from build123d import *

# Parameters (mm, degrees)
SKETCH_1_R          = 13.5
EXTRUDE_1_DEPTH     = 10
SKETCH_2_W          = 12
SKETCH_2_H          = 60
EXTRUDE_2_DEPTH     = 10
SKETCH_3_R          = 10.25
CUT_EXTRUDE_1_DEPTH = 10


with BuildPart() as part:
    # 草图1 → 凸台-拉伸1 (new body)
    with BuildSketch(Plane(origin=(0, 0, 0), x_dir=(1, 0, 0), z_dir=(0, 1, 0))):
        with Locations(Location((0, 0, 0), (0, 0, 270))):
            Circle(SKETCH_1_R)
    extrude(amount=EXTRUDE_1_DEPTH)

    # 草图2 → 凸台-拉伸2 (add)
    with BuildSketch(Plane(origin=(0, 10, 0), x_dir=(1, 0, 0), z_dir=(0, 1, 0))):
        Rectangle(SKETCH_2_W, SKETCH_2_H)
    extrude(amount=-EXTRUDE_2_DEPTH)

    # 草图3 → 切除-拉伸1 (cut)
    with BuildSketch(Plane(origin=(0, 10, 0), x_dir=(1, 0, 0), z_dir=(0, 1, 0))):
        with Locations(Location((0, 0, 0), (0, 0, 270))):
            Circle(SKETCH_3_R)
    extrude(amount=-CUT_EXTRUDE_1_DEPTH, mode=Mode.SUBTRACT)


solid = part.part
The listing builds one solid part. Answer for the finished solid, in the listing's coordinates (mm). A direction names the side the tool comes from. Coordinates: 2 decimals unless noted, no trailing zeros. Order: outer loops, then holes, each group sorted by start corner. A loop starts at its lowest first (then second) coordinate and runs counter-clockwise, first axis right, second up. Notation, with made-up numbers: M 88,67.5 L 115,67.5 A28 cw 115,91.5 Z; hole C -21,-3.75 d4. An arc over 180 degrees is marked long. Use CSV: the item, a comma, the result in double quotes.
Q1. Section A-A (y = 8) is taken. Determine the outline of the cut face in (x, z), then the cut area to 4 significant figures.
Here are the results:
outline,"M -6,-30 L 6,-30 L 6,-12.09 A13.5 ccw 6,12.09 L 6,30 L -6,30 L -6,12.09 A13.5 ccw -6,-12.09 Z; hole C 0,0 d20.5"
area,"649.5 mm2"
Q2. Straight lines are drawn through the part: L1, parallel to X at y = 5, z = 0; L2, parallel to X at y = 2.75, z = -24; L3, parallel to X at y = 2.5, z = -6. For each, find the intervals that lie inside material, in ascending order.
Here are the results:
L1,"-13.5 to -10.25, 10.25 to 13.5"
L2,"-6 to 6"
L3,"-12.09 to -8.31, 8.31 to 12.09"
Q3. Determine the mould class of faces 6 (the cylindrical face through (-10.006, 5.07, -2.222)), 7 (the flat face through (-6, 5, -21)), 8 (the flat face through (9, 0, 6)) for opening direction X: pulls with the +X half, pulls with the -X half, needs draft (parallel to the pull), parting line crosses it, or undercut.
Here are the results:
face 6,"undercut"
face 7,"pulls with the -X half"
face 8,"needs draft"
Q4. Section C-C (z = 0) is taken. Determine the outline of the cut face in (x, y), then the cut area to 3 significant figures.
Here are the results:
outline,"M -13.5,0 L -10.25,0 L -10.25,10 L -13.5,10 Z; M 10.25,0 L 13.5,0 L 13.5,10 L 10.25,10 Z"
area,"65.0 mm2"
Q5. Section D-D (z = -20) is taken. Determine the outline of the cut face in (x, y).
Here are the results:
outline,"M -6,0 L 6,0 L 6,10 L -6,10 Z"
Q6. Given pin 1 Ø2 at (y, z) = (3, -20.5) entering from -X; pin 2 Ø1 at (x, z) = (-6, 10.5) entering from -Y; pin 3 Ø2 at (x, y) = (10, 6) entering from +Z; pin 4 Ø4 at (y, z) = (5.5, -2.5) entering from +X, each flat-ended and moving along its own axis, determine where each tip first touches the part or whether it passes through.
Here are the results:
pin 1,"x = -6"
pin 2,"y = 0"
pin 3,"z = 10.06"
pin 4,"x = 13.49"
Q7. A tool of negligible diameter and unlimited length cuts with its end or side. For faces 1 (the flat face through (6, 5, -21)), 2 (the cylindrical face through (-13.5, 4.9, -0.2)), 3 (the flat face through (-6, 5, 21)), 4 (the flat face through (6, 5, 21)), 5 (the flat face through (9, 10, 6)), from which of +Z, -Z, +X, -X, +Y, -Y can it reach the whole face along a straight path? Write none if from no direction.
Here are the results:
face 1,"-Z, +X, +Y, -Y"
face 2,"-X, +Y, -Y"
face 3,"+Z, -X, +Y, -Y"
face 4,"+Z, +X, +Y, -Y"
face 5,"+Z, -Z, +X, -X, +Y"
Q8. Section B-B (x = 0) is taken. Determine the outline of the cut face in (y, z), then the cut area to 3 significant figures.
Here are the results:
outline,"M 0,-30 L 10,-30 L 10,-10.25 L 0,-10.25 Z; M 0,10.25 L 10,10.25 L 10,30 L 0,30 Z"
area,"395 mm2"
